CAD build for the part. Positions are in the model's coordinates, mm. A direction names the side the tool comes from. Give positions to 0.01 mm unless a question says otherwise; leave off trailing zeros. Write each loop counter-clockwise with the first axis right and the second up, starting at its lowest first coordinate (ties: lowest second). Pieces come first, ordered by that corner, then holes. Notation, with made-up numbers: (32.25, -23) -> (75.25, -23) arc R19 cw to (75.25, -6) -> close; hole circle Ø1 at (-18.5, 68). An arc over 180 degrees is marked (long way). Use one line per item in the form item = value. Start each with the question number.
from build123d import *

# Parameters (mm, degrees)
BOSS_EXTRUDE1_DEPTH = 2
FILLET1_R           = 5
SKETCH2_R           = 1.5
CUT_EXTRUDE1_DEPTH  = 68.426998807
FILLET2_R           = 1


with BuildPart() as part:
    # Sketch1 → Boss-Extrude1 (new body)
    with BuildSketch(Plane(origin=(0, 0, 0), x_dir=(1, 0, 0), z_dir=(0, 1, 0))):
        Polygon((0, 0), (10, 0), (10, 31.741283677), (9.083107298, 36.656495551), (5.221289447, 39.832399027), (1.339003771, 54.321286421), (5.380096521, 58.756325247), (4.088254713, 66.65133283), (-1.911745287, 66.65133283), (-5.952838037, 62.216294005), (0, 40), align=None)
    extrude(amount=BOSS_EXTRUDE1_DEPTH)

    # Fillet1
    fillet1_edges = [part.edges().sort_by_distance(p)[0] for p in [
        (10, 1, 0),
        (0, 1, 0),
    ]]
    fillet(fillet1_edges, radius=FILLET1_R - 0.0001)  # a hair under: the kernel refuses the full size

    # Sketch2 → Cut-Extrude1 (cut, through all)
    with BuildSketch(Plane(origin=(0, 2, 0), x_dir=(1, 0, 0), z_dir=(0, 1, 0))):
        with Locations(Location((0.137851025, 62.574617084, 0), (0, 0, 270))):
            Circle(SKETCH2_R)
        with Locations(Location((5, 5, 0), (0, 0, 270))):
            Circle(SKETCH2_R)
        with Locations(Location((5, 35, 0), (0, 0, 270))):
            Circle(SKETCH2_R)
    extrude(amount=-CUT_EXTRUDE1_DEPTH, mode=Mode.SUBTRACT)

    # Fillet2
    fillet2_edges = [part.edges().sort_by_distance(p)[0] for p in [
        (9.083107298, 1, -36.656495551),
        (10, 1, -31.741283677),
        (0, 1, -40),
        (-5.952838037, 1, -62.216294005),
        (-1.911745287, 1, -66.65133283),
        (1.339003771, 1, -54.321286421),
        (5.221289447, 1, -39.832399027),
    ]]
    fillet(fillet2_edges, radius=FILLET2_R)


solid = part.part
1) Cut at A-A (y = 0.9). State how many separate pieces and enclosed holes the cut face has, and give its area (3 significant figures).
2) Wall check: line 1 along Z through (x, y) = (5.5, 1.9); line 2 along X through (y, z) = (0.6, -5); line 3 along X through (y, z) = (1.3, -29). Give the ranges that are in metal, low to high. Write a range as from..to.
3) 3-axis set-ups, long thin cutter, end or side, ignore diameter. For faces 1 (the face through (3.335, 0.986, -46.872)), 2 (the face through (0, 1, -23)), 3 (the face through (4.743, 0.986, -62.649)): which of +Z, -Z, +X, -X, +Y, -Y reach the whole face in a straight line?
4) Cut at B-B (z = -35). Give the cut face in (x, y).
5) Two-plate mould, pull along X, no slides. Class faces 4 (the face through (-0.44, 1.01, -61.19)), 5 (the face through (8, 1, -1)), 6 (the face through (-2.963, 0.986, -51.059)), 7 (the face through (4.1, 1, -36.2)): released by +X, released by -X, zero draft, split by the parting line, or undercut.
6) Cut at C-C (x = 7.5). Give the cut face in (y, z).
7) Pin check, flat tip, straight feed: pin 1 (1 mm diameter, centred on y = 1.5, z = -30, fed in from -X). Stop position of the tip, or through.
Final values:
q1.separate_pieces = 1
q1.enclosed_holes = 3
q1.area = 538 mm^2
q2.line_1 = -39.6..-36.41, -33.59..-6.41, -3.59..-0.03
q2.line_2 = 0..3.5, 6.5..10
q2.line_3 = 0..10
q3.face_1 = +X, +Y, -Y
q3.face_2 = +Z, -X, +Y, -Y
q3.face_3 = -Z, +X, +Y, -Y
q4.outline = (0, 0) -> (3.5, 0) -> (3.5, 2) -> (0, 2) -> close; (6.5, 0) -> (9.39, 0) -> (9.39, 2) -> (6.5, 2) -> close
q5.face_4 = undercut
q5.face_5 = released by +X
q5.face_6 = released by -X
q5.face_7 = undercut
q6.outline = (0, -37.96) -> (2, -37.96) -> (2, -0.67) -> (0, -0.67) -> close
q7.pin_1 = 0
